For this review, take the finished solid that the model builds, in its own axes (mm). A direction names the side the tool comes from. Give positions to 0.01 mm unless a question says otherwise; leave off trailing zeros. Order: outer loops, then holes, each group sorted by start corner. A loop starts at its lowest first (then second) coordinate and runs counter-clockwise, first axis right, second up. Notation, with made-up numbers: (70, 73) - (118, 73) arc R25 ccw to (118, 101) - close; hole circle Ø7 at (21.25, 18). An arc over 180 degrees is marked (long way). Use a Markdown table: item, result. Add a question column.
1) Wall thickness on L1, parallel to Y at x = 86, z = -238.5; L2, parallel to X at y = 57, z = -117.5; L3, parallel to X at y = 22.5, z = -146: over which ranges is each line inside the solid? List them lowest first.
2) We need section D-D on x = 302.5. Write out the cut boundary in (y, z), then the cut area to 3 significant figures.
3) We need section C-C on x = 12.5. Write out the cut boundary in (y, z), then the cut area to 3 significant figures.
4) We need section B-B on z = -203.5. Write out the cut boundary in (x, y) (3 decimals).
5) Clearance check with flat-ended pins moving along their axes: P1, Ø3, axis at x = 281, z = -252.5, coming from the -Y side; P2, Ø4, axis at y = 37.5, z = -159.5, coming from the -X side; P3, Ø25, axis at x = 190.5, z = -171, coming from the +Y side; P4, Ø22, axis at y = 10, z = -279.5, coming from the -X side. State where each tip first meets the part, or that it passes through.
6) Machinability: for faces 4 (the face through (0, 10, -282)), 5 (the face through (193, 45, -185)), 6 (the face through (330, 35, -162.5)), which of the approach directions +Z, -Z, +X, -X, +Y, -Y give a long, thin tool a straight path to every point of the face, cutting with its end or side? Answer none if there is none.
7) We need section A-A on y = 12. Write out the cut boundary in (x, z).
8) Mouldability with a two-part tool opening along X and no side actions: class faces 1 (the face through (25, 10, -70)), 2 (the face through (259, 70, -161)), 3 (the face through (370, 10, -162)) as released by +X, released by -X, zero draft, split by the parting line, or undercut.
```python
from build123d import *

# Parameters (mm, degrees)
BOSS_EXTRUDE1_DEPTH     = 20
CUT_EXTRUDE1_DEPTH      = 490.591666596
CUT_EXTRUDE1_DEPTH_BACK = 490.591666596
SKETCH2_W               = 20
SKETCH2_H               = 5
SKETCH3_W               = 200
SKETCH3_H               = 200
SKETCH3_W_2             = 50
SKETCH3_H_2             = 50
BOSS_EXTRUDE2_DEPTH     = 50
SKETCH4_W               = 20
SKETCH4_H               = 5
CUT_EXTRUDE2_DEPTH      = 495.165964024


with BuildPart() as part:
    # Sketch1 → Boss-Extrude1 (new body)
    with BuildSketch(Plane(origin=(0, 0, 0), x_dir=(1, 0, 0), z_dir=(0, 1, 0))):
        Polygon((0, 75), (50, 35), (0, 105), (0, 215), (-50, 175), (0, 245), (0, 320), (370, 320), (370, 0), (0, 0), align=None)
    extrude(amount=BOSS_EXTRUDE1_DEPTH)

    # Sketch2 → Cut-Extrude1 (cut, two sides: drawn at the far end of the back side and taken through both)
    with BuildSketch(Plane.XZ.offset(-CUT_EXTRUDE1_DEPTH_BACK)):
        with Locations((330, -160)):
            Rectangle(SKETCH2_W, SKETCH2_H)
    extrude(amount=CUT_EXTRUDE1_DEPTH + CUT_EXTRUDE1_DEPTH_BACK, mode=Mode.SUBTRACT)

    # Sketch3 → Boss-Extrude2 (add)
    with BuildSketch(Plane(origin=(0, 20, 0), x_dir=(1, 0, 0), z_dir=(0, 1, 0))):
        with Locations((260, 160)):
            Rectangle(SKETCH3_W, SKETCH3_H)
        with Locations((193.4, 160)):
            Rectangle(SKETCH3_W_2, SKETCH3_H_2, mode=Mode.SUBTRACT)
    extrude(amount=BOSS_EXTRUDE2_DEPTH)

    # Sketch4 → Cut-Extrude2 (cut, through all)
    with BuildSketch(Plane.XZ):
        with Locations((330, -160)):
            Rectangle(SKETCH4_W, SKETCH4_H)
    extrude(amount=-CUT_EXTRUDE2_DEPTH, mode=Mode.SUBTRACT)


solid = part.part
```
Checked values:
| question | item | result |
|---|---|---|
| 1 | L1 | 0 to 20 |
| 1 | L2 | 160 to 360 |
| 1 | L3 | 160 to 168.4, 218.4 to 360 |
| 2 | outline | (0, -320) - (20, -320) - (20, -260) - (70, -260) - (70, -60) - (20, -60) - (20, 0) - (0, 0) - close |
| 2 | area | 16,400 mm² |
| 3 | outline | (0, -320) - (20, -320) - (20, -87.5) - (0, -87.5) - close; (0, -65) - (20, -65) - (20, 0) - (0, 0) - close |
| 3 | area | 5,950 mm² |
| 4 | outline | (-29.643, 0) - (-14.375, 0) - (-14.375, 20) - (-29.643, 20) - close; (0, 0) - (370, 0) - (370, 20) - (360, 20) - (360, 70) - (160, 70) - (160, 20) - (0, 20) - close |
| 5 | P1 | y = 0 |
| 5 | P2 | x = 160 |
| 5 | P3 | y = 20 |
| 5 | P4 | x = 0 |
| 6 | face 4 | -Z, -X, +Y, -Y |
| 6 | face 5 | +Y |
| 6 | face 6 | +Y, -Y |
| 7 | outline | (-50, -175) - (0, -245) - (0, -320) - (370, -320) - (370, 0) - (0, 0) - (0, -75) - (50, -35) - (0, -105) - (0, -215) - close; hole (320, -162.5) - (340, -162.5) - (340, -157.5) - (320, -157.5) - close |
| 8 | face 1 | undercut |
| 8 | face 2 | zero draft |
| 8 | face 3 | released by +X |
